Geometry check sheet. Reference: the model listing, model coordinates, mm. Face numbers are marked on the shaded views. A direction names the side the tool comes from. Round coordinates to 2 decimals unless told otherwise and drop trailing zeros. Loops run counter-clockwise (first coordinate to the right, second up) from the corner with the lowest first, then second, coordinate; pieces in that order, holes last. Notation, with made-up numbers: (-34, 76.5) - (25, 76.5) arc R23 cw to (25, 115.5) - close; hole circle Ø8 at (12, 54.25). An arc over 180 degrees is marked (long way). Answer as CSV lines item,"result". Start each with the question number.
1) Cross-section at C-C on x = 234.5. State how many separate pieces and enclosed holes the cut face has, and give its area (3 significant figures).
2) Cross-section at D-D on z = 38.75. Record the boundary of the cut face in (x, y) (3 decimals).
3) Draft check along X on the marked faces 1, 2 and 3. Enter one of: released by +X, released by -X, zero draft, split by the parting line, or undercut.
4) Cross-section at A-A on y = 482. Record the boundary of the cut face in (x, z), and give its area (3 significant figures).
5) Thickness scan on line 1 along X through (y, z) = (484.5, 29.75); line 2 along Y through (x, z) = (236.5, 33.5); line 3 along Y through (x, z) = (241.75, 31.25). Record the ranges inside material, lowest first.
6) Depth check by flat-ended pin: P1, Ø3.5, axis at x = 239, z = 30, coming from the -Y side; P2, Ø1.8, axis at x = 239, y = 467.27, coming from the +Z side; P3, Ø6, axis at y = 482.5, z = 28, coming from the +X side. Enter the tip coordinate at first touch or a pass-through.
7) Access from +Z, -Z, +X, -X, +Y, -Y to the whole of each face (thin tool, end or side, straight path). Record for the marked faces 4, 5 and 6.
from build123d import *

# Parameters (mm, degrees)
SKETCH1_W           = 14
SKETCH1_H           = 34
BOSS_EXTRUDE1_DEPTH = 7
SKETCH2_R           = 1
SKETCH2_W           = 12
SKETCH2_H           = 24.4
CUT_EXTRUDE1_DEPTH  = 555.564285541
SKETCH3_W           = 14
SKETCH3_H           = 5
BOSS_EXTRUDE2_DEPTH = 5
SKETCH4_W           = 14
SKETCH4_H           = 3
BOSS_EXTRUDE3_DEPTH = 5
FILLET1_R           = 1.5
FILLET2_R           = 0.8
SKETCH5_R           = 1
CUT_EXTRUDE2_DEPTH  = 7
SKETCH6_R           = 1
CUT_EXTRUDE3_DEPTH  = 252.483055086


with BuildPart() as part:
    # Sketch1 → Boss-Extrude1 (new body)
    with BuildSketch(Plane.XY.offset(25)):
        with Locations((238.952994655, 479.990614818)):
            Rectangle(SKETCH1_W, SKETCH1_H)
    extrude(amount=BOSS_EXTRUDE1_DEPTH)

    # Sketch2 → Cut-Extrude1 (cut, through all)
    with BuildSketch(Plane.XY.offset(32)):
        with Locations((238.935079192, 495.003072258)):
            Circle(SKETCH2_R)
        with Locations((239, 481.000012207)):
            Rectangle(SKETCH2_W, SKETCH2_H)
    extrude(amount=-CUT_EXTRUDE1_DEPTH, mode=Mode.SUBTRACT)

    # Sketch3 → Boss-Extrude2 (add)
    with BuildSketch(Plane.XY.offset(32)):
        with Locations((239, 465.5)):
            Rectangle(SKETCH3_W, SKETCH3_H)
    extrude(amount=BOSS_EXTRUDE2_DEPTH)

    # Sketch4 → Boss-Extrude3 (add)
    with BuildSketch(Plane.XY.offset(37)):
        with Locations((239, 464.446662177)):
            Rectangle(SKETCH4_W, SKETCH4_H)
    extrude(amount=BOSS_EXTRUDE3_DEPTH)

    # Fillet1
    fillet1_edges = [part.edges().sort_by_distance(p)[0] for p in [
        (232, 464.446662177, 42),
        (246, 464.446662177, 42),
        (231.952994655, 496.990614818, 28.5),
        (245.952994655, 496.990614818, 28.5),
    ]]
    fillet(fillet1_edges, radius=FILLET1_R)

    # Fillet2
    fillet2_edges = [part.edges().sort_by_distance(p)[0] for p in [
        (239, 468, 37),
        (239, 465.946662177, 37),
    ]]
    fillet(fillet2_edges, radius=FILLET2_R)

    # Sketch5 → Cut-Extrude2 (cut)
    with BuildSketch(Plane(origin=(0, 0, 25), x_dir=(-1, 0, 0), z_dir=(0, 0, -1))):
        with Locations((-238.99635452, 467.272454622)):
            Circle(SKETCH5_R)
    extrude(amount=-CUT_EXTRUDE2_DEPTH, mode=Mode.SUBTRACT)

    # Sketch6 → Cut-Extrude3 (cut, through all)
    with BuildSketch(Plane(origin=(0, 465.946662177, 0), x_dir=(1, 0, 0), z_dir=(0, 1, 0))):
        with Locations(Location((234.951502539, -39.341225233, 0), (0, 0, 270))):
            Circle(SKETCH6_R)
        with Locations(Location((242.951502539, -39.341225233, 0), (0, 0, 270))):
            Circle(SKETCH6_R)
    extrude(amount=-CUT_EXTRUDE3_DEPTH, mode=Mode.SUBTRACT)


solid = part.part
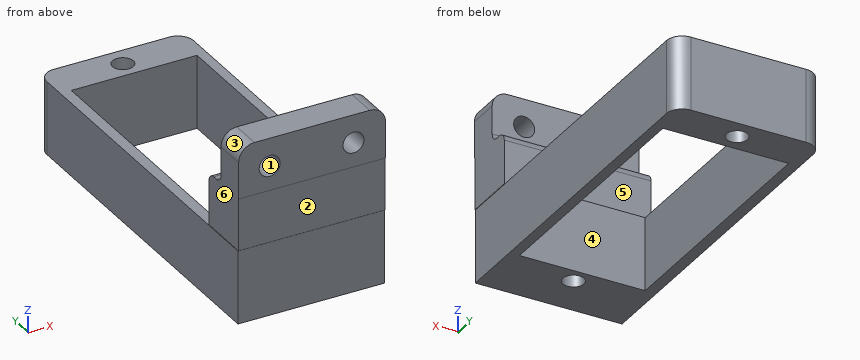
Answer block:
1,separate pieces,"3"
1,enclosed holes,"0"
1,area,"102 mm^2"
2,outline,"(232, 462.947) - (234.145, 462.947) - (234.145, 465.947) - (232, 465.947) - close; (235.758, 462.947) - (242.145, 462.947) - (242.145, 465.947) - (235.758, 465.947) - close; (243.758, 462.947) - (246, 462.947) - (246, 465.947) - (243.758, 465.947) - close"
3,face 1,"undercut"
3,face 2,"zero draft"
3,face 3,"released by -X"
4,outline,"(231.95, 25) - (233, 25) - (233, 32) - (231.95, 32) - close; (245, 25) - (245.95, 25) - (245.95, 32) - (245, 32) - close"
4,area,"14.0 mm^2"
5,line 1,"x = 231.95 to 233, 245 to 245.95"
5,line 2,"y = 463 to 468"
5,line 3,"y = 462.99 to 468.8, 493.2 to 496.99"
6,P1,"stops at y = 462.99"
6,P2,"stops at z = 37.09"
6,P3,"stops at x = 245.95"
7,face 4,"+Z, -Z"
7,face 5,"+Z, +X, -X, +Y"
7,face 6,"+Z, -X, +Y, -Y"
